from build123d import *

# Parameters (mm, degrees)
SKETCH1_R           = 1.55
BOSS_EXTRUDE3_DEPTH = 3.175


with BuildPart() as part:
    # Sketch1 → Boss-Extrude3 (new body)
    with BuildSketch(Plane(origin=(0, 0, 0), x_dir=(0, 0, -1), z_dir=(1, 0, 0))):
        with BuildLine():
            Line((3.75, -3.307189139), (3.75, -81.692810861))
            ThreePointArc((3.75, -81.692810861), (0, -90), (-3.75, -81.692810861))
            Line((-3.75, -81.692810861), (-3.75, -3.307189139))
            ThreePointArc((-3.75, -3.307189139), (0, 5), (3.75, -3.307189139))
        make_face()
        with Locations((0, -85)):
            Circle(SKETCH1_R, mode=Mode.SUBTRACT)
        with BuildLine():
            Line((-1.754399331, 1.096511265), (-2.099123622, 1.110992809))
            ThreePointArc((-2.099123622, 1.110992809), (-2.186107384, 0.928202298), (-2.257209306, 0.738668497))
            Line((-2.257209306, 0.738668497), (-2.007373532, 0.500704976))
            Line((-2.007373532, 0.500704976), (-2.339700857, 0.407952078))
            ThreePointArc((-2.339700857, 0.407952078), (-2.365941957, 0.207228511), (-2.374994738, 0.004999452))
            Line((-2.374994738, 0.004999452), (-2.063852025, -0.144113805))
            Line((-2.063852025, -0.144113805), (-2.351251872, -0.335021845))
            ThreePointArc((-2.351251872, -0.335021845), (-2.314181647, -0.534030246), (-2.260299137, -0.729158975))
            Line((-2.260299137, -0.729158975), (-1.918306302, -0.774825723))
            Line((-1.918306302, -0.774825723), (-2.13264597, -1.045201495))
            ThreePointArc((-2.13264597, -1.045201495), (-2.035893114, -1.223014403), (-1.924349708, -1.39194224))
            Line((-1.924349708, -1.39194224), (-1.584983392, -1.329692301))
            Line((-1.584983392, -1.329692301), (-1.705281823, -1.65306954))
            ThreePointArc((-1.705281823, -1.65306954), (-1.558317177, -1.792281388), (-1.400031522, -1.918472501))
            Line((-1.400031522, -1.918472501), (-1.096511265, -1.754399331))
            Line((-1.096511265, -1.754399331), (-1.110992809, -2.099123622))
            ThreePointArc((-1.110992809, -2.099123622), (-0.928202298, -2.186107384), (-0.738668497, -2.257209306))
            Line((-0.738668497, -2.257209306), (-0.500704976, -2.007373532))
            Line((-0.500704976, -2.007373532), (-0.407952078, -2.339700857))
            ThreePointArc((-0.407952078, -2.339700857), (-0.207228511, -2.365941957), (-0.004999452, -2.374994738))
            Line((-0.004999452, -2.374994738), (0.144113805, -2.063852025))
            Line((0.144113805, -2.063852025), (0.335021845, -2.351251872))
            ThreePointArc((0.335021845, -2.351251872), (0.534030246, -2.314181647), (0.729158975, -2.260299137))
            Line((0.729158975, -2.260299137), (0.774825723, -1.918306302))
            Line((0.774825723, -1.918306302), (1.045201495, -2.13264597))
            ThreePointArc((1.045201495, -2.13264597), (1.223014403, -2.035893114), (1.39194224, -1.924349708))
            Line((1.39194224, -1.924349708), (1.329692301, -1.584983392))
            Line((1.329692301, -1.584983392), (1.65306954, -1.705281823))
            ThreePointArc((1.65306954, -1.705281823), (1.792281388, -1.558317177), (1.918472501, -1.400031522))
            Line((1.918472501, -1.400031522), (1.754399331, -1.096511265))
            Line((1.754399331, -1.096511265), (2.099123622, -1.110992809))
            ThreePointArc((2.099123622, -1.110992809), (2.186107384, -0.928202298), (2.257209306, -0.738668497))
            Line((2.257209306, -0.738668497), (2.007373532, -0.500704976))
            Line((2.007373532, -0.500704976), (2.339700857, -0.407952078))
            ThreePointArc((2.339700857, -0.407952078), (2.365941957, -0.207228511), (2.374994738, -0.004999452))
            Line((2.374994738, -0.004999452), (2.063852025, 0.144113805))
            Line((2.063852025, 0.144113805), (2.351251872, 0.335021845))
            ThreePointArc((2.351251872, 0.335021845), (2.314181647, 0.534030246), (2.260299137, 0.729158975))
            Line((2.260299137, 0.729158975), (1.918306302, 0.774825723))
            Line((1.918306302, 0.774825723), (2.13264597, 1.045201495))
            ThreePointArc((2.13264597, 1.045201495), (2.035893114, 1.223014403), (1.924349708, 1.39194224))
            Line((1.924349708, 1.39194224), (1.584983392, 1.329692301))
            Line((1.584983392, 1.329692301), (1.705281823, 1.65306954))
            ThreePointArc((1.705281823, 1.65306954), (1.558317177, 1.792281388), (1.400031522, 1.918472501))
            Line((1.400031522, 1.918472501), (1.096511265, 1.754399331))
            Line((1.096511265, 1.754399331), (1.110992809, 2.099123622))
            ThreePointArc((1.110992809, 2.099123622), (0.928202298, 2.186107384), (0.738668497, 2.257209306))
            Line((0.738668497, 2.257209306), (0.500704976, 2.007373532))
            Line((0.500704976, 2.007373532), (0.407952078, 2.339700857))
            ThreePointArc((0.407952078, 2.339700857), (0.207228511, 2.365941957), (0.004999452, 2.374994738))
            Line((0.004999452, 2.374994738), (-0.144113805, 2.063852025))
            Line((-0.144113805, 2.063852025), (-0.335021845, 2.351251872))
            ThreePointArc((-0.335021845, 2.351251872), (-0.534030246, 2.314181647), (-0.729158975, 2.260299137))
            Line((-0.729158975, 2.260299137), (-0.774825723, 1.918306302))
            Line((-0.774825723, 1.918306302), (-1.045201495, 2.13264597))
            ThreePointArc((-1.045201495, 2.13264597), (-1.223014403, 2.035893114), (-1.39194224, 1.924349708))
            Line((-1.39194224, 1.924349708), (-1.329692301, 1.584983392))
            Line((-1.329692301, 1.584983392), (-1.65306954, 1.705281823))
            ThreePointArc((-1.65306954, 1.705281823), (-1.792281388, 1.558317177), (-1.918472501, 1.400031522))
            Line((-1.918472501, 1.400031522), (-1.754399331, 1.096511265))
        make_face(mode=Mode.SUBTRACT)
    extrude(amount=BOSS_EXTRUDE3_DEPTH)


solid = part.part
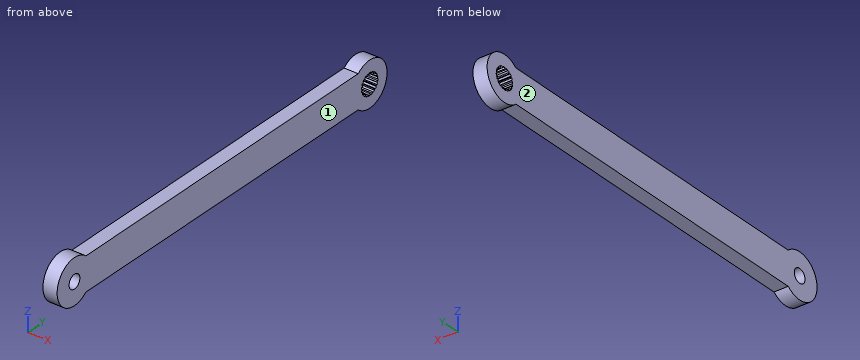
The listing builds one solid part. Answer for the finished solid, in the listing's coordinates (mm). Face numbers are marked on the shaded views. Coordinates: 2 decimals unless noted, no trailing zeros. Order: outer loops, then holes, each group sorted by start corner. A loop starts at its lowest first (then second) coordinate and runs counter-clockwise, first axis right, second up. Notation, with made-up numbers: (48, 12.25) -> (93, 12.25) arc R18 cw to (93, 39.25) -> close; hole circle Ø1 at (59.25, 63.5). An arc over 180 degrees is marked (long way). Answer in a Markdown table with one row per item. Add a question column.
Item 1: Find section A-A (y = -85). Write down the section's boundary in (x, z) (3 decimals).
Item 2: Determine the mould class of the marked faces 1 and 2 for opening direction X: +X half, -X half, draft (parallel to the pull), parting line (faces both ways), or undercut.
Item 3: Find the intervals of material crossed by L1, parallel to Y at x = 1.65, z = 0; L2, parallel to Z at x = 1.4, y = -85; L3, parallel to Z at x = 1.15, y = -19, in increasing order. Write a range as from..to.
Item 4: Each of these flat-tipped pins is pushed along its axis until it touches: P1, Ø1.5, axis at x = 1, y = -34, coming from the -Z side; P2, Ø1.6, axis at x = 1, y = -53, coming from the +Z side; P3, Ø1.9, axis at y = -85, z = 0, coming from the -X side. Where does it stop, or does it pass through?
Item 5: Find section C-C (y = -64). Write down the section's boundary in (x, z) (3 decimals).
Item 6: Find section B-B (x = 0.95). State how many separate pieces and enclosed holes the cut face has, then the cut area to 3 significant figures.
Result set:
| question | item | result |
|---|---|---|
| 1 | outline | (0, -5) -> (3.175, -5) -> (3.175, -1.55) -> (0, -1.55) -> close; (0, 1.55) -> (3.175, 1.55) -> (3.175, 5) -> (0, 5) -> close |
| 2 | face 1 | +X half |
| 2 | face 2 | -X half |
| 3 | L1 | y = -90..-86.55, -83.45..-2.36, 2.36..5 |
| 3 | L2 | z = -5..-1.55, 1.55..5 |
| 3 | L3 | z = -3.75..3.75 |
| 4 | P1 | stops at z = -3.75 |
| 4 | P2 | stops at z = 3.75 |
| 4 | P3 | passes through |
| 5 | outline | (0, -3.75) -> (3.175, -3.75) -> (3.175, 3.75) -> (0, 3.75) -> close |
| 6 | separate pieces | 1 |
| 6 | enclosed holes | 2 |
| 6 | area | 703 mm² |
